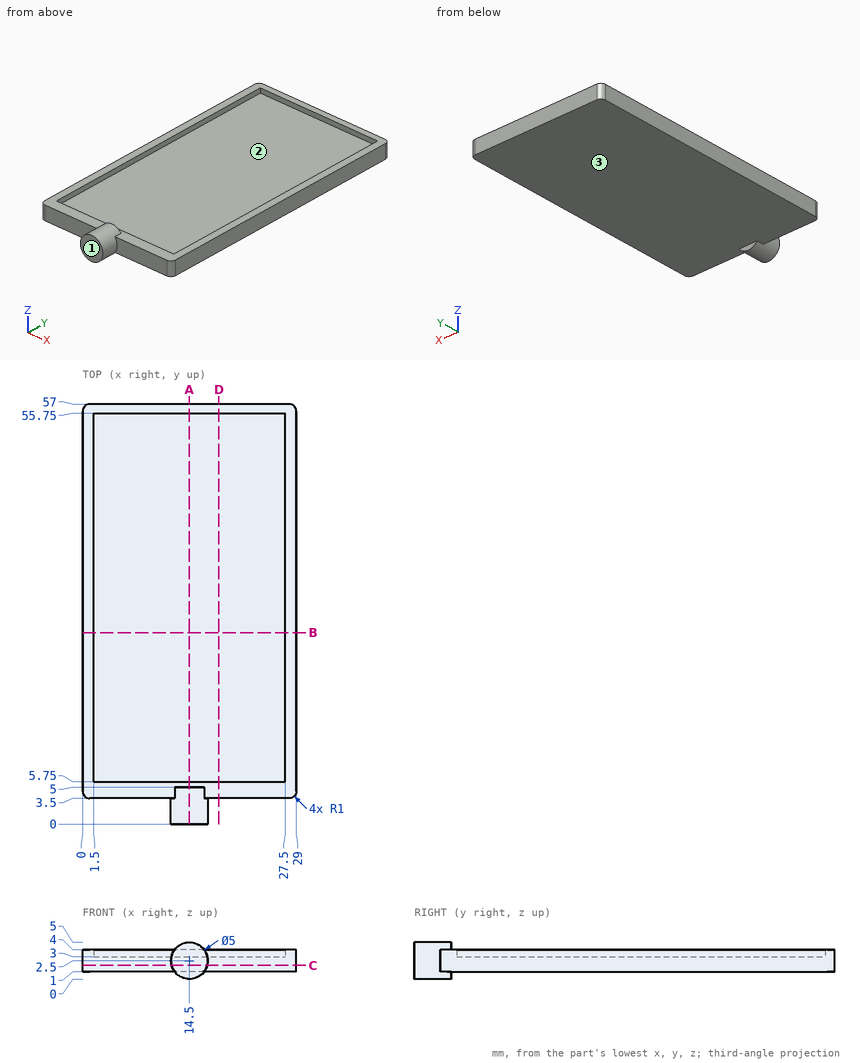
Part print with two shaded views. Sizes in mm from the minimum x, y, z corner. Coordinates: 2 decimals unless noted, no trailing zeros. Write each loop counter-clockwise with the first axis right and the second up, starting at its lowest first coordinate (ties: lowest second). Pieces come first, ordered by that corner, then holes. Notation, with made-up numbers: (86, -32) - (126, -32) arc R20 ccw to (126, -9) - close; hole circle Ø3 at (70.25, 64.25). An arc over 180 degrees is marked (long way). Put each result on its own line as item: value.
1. Band-saw the part on B-B (y = 26). Write the cut outline in (x, z).
Final values:
outline: (0, 1) - (29, 1) - (29, 4) - (27.5, 4) - (27.5, 3) - (1.5, 3) - (1.5, 4) - (0, 4) - close
2. Band-saw the part on A-A (x = 14.5). Write the cut outline in (y, z).
Final values:
outline: (0, 0) - (5, 0) - (5, 1) - (57, 1) - (57, 4) - (55.75, 4) - (55.75, 3) - (5.75, 3) - (5.75, 4) - (5, 4) - (5, 5) - (0, 5) - close
3. Band-saw the part on C-C (z = 1.85). Write the cut outline in (x, y).
Final values:
outline: (0, 4.5) arc R1 ccw to (1, 3.5) - (12.09, 3.5) - (12.09, 0) - (16.91, 0) - (16.91, 3.5) - (28, 3.5) arc R1 ccw to (29, 4.5) - (29, 56) arc R1 ccw to (28, 57) - (1, 57) arc R1 ccw to (0, 56) - close
4. Flat gauge pins, fed straight in: pin 1 Ø1.5 at (x, z) = (8, 3) entering from -Y; pin 2 Ø0.5 at (x, z) = (14.5, 0.5) entering from +Y; pin 3 Ø8 at (x, y) = (20.5, 41) entering from +Z. Where does each tip first touch, or does it go through?
Final values:
pin 1: stops at y = 3.5
pin 2: stops at y = 5
pin 3: stops at z = 3
5. Two-plate mould, pull along Y, no slides. Class the marked faces 1, 2 and 3: +Y half, -Y half, draft (parallel to the pull), parting line (faces both ways), or undercut.
Final values:
face 1: -Y half
face 2: undercut
face 3: draft
6. Probe line 1 along X through (y, z) = (6.5, 3.3); line 2 along Y through (x, z) = (17.5, 3.9); line 3 along Z through (x, y) = (22.25, 43.5). List the from-to ranges inside material, lowest first. Write a range as [from, to].
Final values:
line 1: x = [0, 1.5], [27.5, 29]
line 2: y = [3.5, 5.75], [55.75, 57]
line 3: z = [1, 3]
7. Band-saw the part on D-D (x = 18.5). Write the cut outline in (y, z).
Final values:
outline: (3.5, 1) - (57, 1) - (57, 4) - (55.75, 4) - (55.75, 3) - (5.75, 3) - (5.75, 4) - (3.5, 4) - close
